Build history of the part. All positions in model axes, mm. A direction names the side the tool comes from. Give positions to 0.01 mm unless a question says otherwise; leave off trailing zeros. Order: outer loops, then holes, each group sorted by start corner. A loop starts at its lowest first (then second) coordinate and runs counter-clockwise, first axis right, second up. Notation, with made-up numbers: M 48,3 L 82,3 A25 ccw 82,26 Z; hole C 69,-8.75 d5. An arc over 180 degrees is marked long. One line per item, written item: value.
from build123d import *

# Parameters (mm, degrees)
SZKIC1_W                    = 121
SZKIC1_H                    = 24
SZKIC1_R                    = 7.5
DODANIE_WYCI_GNI_CIE1_DEPTH = 3
SZKIC2_W                    = 121
SZKIC2_H                    = 24
SZKIC2_W_2                  = 39
SZKIC2_H_2                  = 20
DODANIE_WYCI_GNI_CIE2_DEPTH = 2
SZKIC3_W                    = 10
SZKIC3_H                    = 21
SZKIC3_W_2                  = 18
DODANIE_WYCI_GNI_CIE3_DEPTH = 5
SZKIC5_W                    = 18
SZKIC5_H                    = 9
DODANIE_WYCI_GNI_CIE4_DEPTH = 2.5
WYTNIJ_WYCI_GNI_CIE1_REACH  = 103.983
SZKIC6_R                    = 1.75
WYTNIJ_WYCI_GNI_CIE2_START  = -1.5
SZKIC7_R                    = 3.75
SZKIC7_R_2                  = 1.75
WYTNIJ_WYCI_GNI_CIE2_DEPTH  = 1.5
WYTNIJ_WYCI_GNI_CIE4_DEPTH  = 1.5
ZAOKR_GLENIE1_R             = 1.5
SZKIC10_W                   = 10
SZKIC10_H                   = 7.5
SZKIC10_W_2                 = 18
WYTNIJ_WYCI_GNI_CIE5_DEPTH  = 0.2
SZKIC11_W                   = 121
SZKIC11_H                   = 1.5
DODANIE_WYCI_GNI_CIE5_DEPTH = 45
SFAZOWANIE1_SIZE            = 1
SFAZOWANIE2_SIZE            = 1


with BuildPart() as part:
    # Szkic1 → Dodanie-wyciągnięcie1 (new body)
    with BuildSketch(Plane.XY):
        with Locations((40, 0)):
            Rectangle(SZKIC1_W, SZKIC1_H)
        Circle(SZKIC1_R, mode=Mode.SUBTRACT)
        with Locations((80, 0)):
            Circle(SZKIC1_R, mode=Mode.SUBTRACT)
    extrude(amount=DODANIE_WYCI_GNI_CIE1_DEPTH)

    # Szkic2 → Dodanie-wyciągnięcie2 (add)
    with BuildSketch(Plane.XY.offset(3)):
        with Locations((40, 0)):
            Rectangle(SZKIC2_W, SZKIC2_H)
        with Locations((9, 0)):
            Rectangle(SZKIC2_W_2, SZKIC2_H_2, mode=Mode.SUBTRACT)
        with Locations((71, 0)):
            Rectangle(SZKIC2_W_2, SZKIC2_H_2, mode=Mode.SUBTRACT)
    extrude(amount=DODANIE_WYCI_GNI_CIE2_DEPTH)

    # Szkic3 → Dodanie-wyciągnięcie3 (add)
    with BuildSketch(Plane.XY.offset(5)):
        with Locations((-15.5, 0)):
            Rectangle(SZKIC3_W, SZKIC3_H)
        with Locations((40, 0)):
            Rectangle(SZKIC3_W_2, SZKIC3_H)
        with Locations((95.5, 0)):
            Rectangle(SZKIC3_W, SZKIC3_H)
    extrude(amount=DODANIE_WYCI_GNI_CIE3_DEPTH)

    # Szkic5 → Dodanie-wyciągnięcie4 (add)
    with BuildSketch(Plane.XY.offset(10)):
        Polygon((-20.5, 10.5), (-10.5, 10.5), (-10.5, 1.5), (-19, 1.5), (-19, -1.5), (-10.5, -1.5), (-10.5, -10.5), (-20.5, -10.5), align=None)
        Polygon((90.5, -1.5), (99, -1.5), (99, 1.5), (90.5, 1.5), (90.5, 10.5), (100.5, 10.5), (100.5, -10.5), (90.5, -10.5), align=None)
        with Locations((40, -6)):
            Rectangle(SZKIC5_W, SZKIC5_H)
        with Locations((40, 6)):
            Rectangle(SZKIC5_W, SZKIC5_H)
    extrude(amount=DODANIE_WYCI_GNI_CIE4_DEPTH)

    # Szkic6 → Wytnij-wyciągnięcie1 (cut, up to next)
    with BuildSketch(Plane.XY.offset(12.5), mode=Mode.PRIVATE) as wytnij_wyci_gni_cie1_sk1:
        with Locations((-14.5, 5.45)):
            Circle(SZKIC6_R)
    wytnij_wyci_gni_cie1_tool1 = extrude(wytnij_wyci_gni_cie1_sk1.sketch, amount=-WYTNIJ_WYCI_GNI_CIE1_REACH, mode=Mode.PRIVATE) & part.part
    # Szkic6 → Wytnij-wyciągnięcie1 (cut, up to next)
    with BuildSketch(Plane.XY.offset(12.5), mode=Mode.PRIVATE) as wytnij_wyci_gni_cie1_sk2:
        with Locations((34.5, 5.45)):
            Circle(SZKIC6_R)
    wytnij_wyci_gni_cie1_tool2 = extrude(wytnij_wyci_gni_cie1_sk2.sketch, amount=-WYTNIJ_WYCI_GNI_CIE1_REACH, mode=Mode.PRIVATE) & part.part
    # Szkic6 → Wytnij-wyciągnięcie1 (cut, up to next)
    with BuildSketch(Plane.XY.offset(12.5), mode=Mode.PRIVATE) as wytnij_wyci_gni_cie1_sk3:
        with Locations((34.5, -5.45)):
            Circle(SZKIC6_R)
    wytnij_wyci_gni_cie1_tool3 = extrude(wytnij_wyci_gni_cie1_sk3.sketch, amount=-WYTNIJ_WYCI_GNI_CIE1_REACH, mode=Mode.PRIVATE) & part.part
    # Szkic6 → Wytnij-wyciągnięcie1 (cut, up to next)
    with BuildSketch(Plane.XY.offset(12.5), mode=Mode.PRIVATE) as wytnij_wyci_gni_cie1_sk4:
        with Locations((-14.5, -5.45)):
            Circle(SZKIC6_R)
    wytnij_wyci_gni_cie1_tool4 = extrude(wytnij_wyci_gni_cie1_sk4.sketch, amount=-WYTNIJ_WYCI_GNI_CIE1_REACH, mode=Mode.PRIVATE) & part.part
    # Szkic6 → Wytnij-wyciągnięcie1 (cut, up to next)
    with BuildSketch(Plane.XY.offset(12.5), mode=Mode.PRIVATE) as wytnij_wyci_gni_cie1_sk5:
        with Locations((45.5, 5.45)):
            Circle(SZKIC6_R)
    wytnij_wyci_gni_cie1_tool5 = extrude(wytnij_wyci_gni_cie1_sk5.sketch, amount=-WYTNIJ_WYCI_GNI_CIE1_REACH, mode=Mode.PRIVATE) & part.part
    # Szkic6 → Wytnij-wyciągnięcie1 (cut, up to next)
    with BuildSketch(Plane.XY.offset(12.5), mode=Mode.PRIVATE) as wytnij_wyci_gni_cie1_sk6:
        with Locations((45.5, -5.45)):
            Circle(SZKIC6_R)
    wytnij_wyci_gni_cie1_tool6 = extrude(wytnij_wyci_gni_cie1_sk6.sketch, amount=-WYTNIJ_WYCI_GNI_CIE1_REACH, mode=Mode.PRIVATE) & part.part
    # Szkic6 → Wytnij-wyciągnięcie1 (cut, up to next)
    with BuildSketch(Plane.XY.offset(12.5), mode=Mode.PRIVATE) as wytnij_wyci_gni_cie1_sk7:
        with Locations((94.5, -5.45)):
            Circle(SZKIC6_R)
    wytnij_wyci_gni_cie1_tool7 = extrude(wytnij_wyci_gni_cie1_sk7.sketch, amount=-WYTNIJ_WYCI_GNI_CIE1_REACH, mode=Mode.PRIVATE) & part.part
    # Szkic6 → Wytnij-wyciągnięcie1 (cut, up to next)
    with BuildSketch(Plane.XY.offset(12.5), mode=Mode.PRIVATE) as wytnij_wyci_gni_cie1_sk8:
        with Locations((94.5, 5.45)):
            Circle(SZKIC6_R)
    wytnij_wyci_gni_cie1_tool8 = extrude(wytnij_wyci_gni_cie1_sk8.sketch, amount=-WYTNIJ_WYCI_GNI_CIE1_REACH, mode=Mode.PRIVATE) & part.part
    add(wytnij_wyci_gni_cie1_tool1.solids().sort_by_distance((-14.5, 5.45, 12.5))[0], mode=Mode.SUBTRACT)
    add(wytnij_wyci_gni_cie1_tool2.solids().sort_by_distance((34.5, 5.45, 12.5))[0], mode=Mode.SUBTRACT)
    add(wytnij_wyci_gni_cie1_tool3.solids().sort_by_distance((34.5, -5.45, 12.5))[0], mode=Mode.SUBTRACT)
    add(wytnij_wyci_gni_cie1_tool4.solids().sort_by_distance((-14.5, -5.45, 12.5))[0], mode=Mode.SUBTRACT)
    add(wytnij_wyci_gni_cie1_tool5.solids().sort_by_distance((45.5, 5.45, 12.5))[0], mode=Mode.SUBTRACT)
    add(wytnij_wyci_gni_cie1_tool6.solids().sort_by_distance((45.5, -5.45, 12.5))[0], mode=Mode.SUBTRACT)
    add(wytnij_wyci_gni_cie1_tool7.solids().sort_by_distance((94.5, -5.45, 12.5))[0], mode=Mode.SUBTRACT)
    add(wytnij_wyci_gni_cie1_tool8.solids().sort_by_distance((94.5, 5.45, 12.5))[0], mode=Mode.SUBTRACT)

    # Szkic7 → Wytnij-wyciągnięcie2 (cut)
    # profile 1 of 4: a face of its own
    with BuildSketch(Plane(origin=(0, 0, 0), x_dir=(-1, 0, 0), z_dir=(0, 0, -1)).offset(WYTNIJ_WYCI_GNI_CIE2_START)):
        with Locations((14.5, -5.45)):
            Circle(SZKIC7_R)
        with Locations(Location((14.5, -5.45, 0), (0, 0, 180))):
            Circle(SZKIC7_R_2, mode=Mode.SUBTRACT)
    # profile 2 of 4: a face of its own
    with BuildSketch(Plane(origin=(0, 0, 0), x_dir=(-1, 0, 0), z_dir=(0, 0, -1)).offset(WYTNIJ_WYCI_GNI_CIE2_START)):
        with Locations((14.5, 5.45)):
            Circle(SZKIC7_R)
        with Locations(Location((14.5, 5.45, 0), (0, 0, 180))):
            Circle(SZKIC7_R_2, mode=Mode.SUBTRACT)
    # profile 3 of 4: a face of its own
    with BuildSketch(Plane(origin=(0, 0, 0), x_dir=(-1, 0, 0), z_dir=(0, 0, -1)).offset(WYTNIJ_WYCI_GNI_CIE2_START)):
        with Locations((-94.5, -5.45)):
            Circle(SZKIC7_R)
        with Locations(Location((-94.5, -5.45, 0), (0, 0, 180))):
            Circle(SZKIC7_R_2, mode=Mode.SUBTRACT)
    # profile 4 of 4: a face of its own
    with BuildSketch(Plane(origin=(0, 0, 0), x_dir=(-1, 0, 0), z_dir=(0, 0, -1)).offset(WYTNIJ_WYCI_GNI_CIE2_START)):
        with Locations((-94.5, 5.45)):
            Circle(SZKIC7_R)
        with Locations(Location((-94.5, 5.45, 0), (0, 0, 180))):
            Circle(SZKIC7_R_2, mode=Mode.SUBTRACT)
    extrude(amount=WYTNIJ_WYCI_GNI_CIE2_DEPTH, mode=Mode.SUBTRACT)

    # Szkic9 → Wytnij-wyciągnięcie4 (cut)
    with BuildSketch(Plane(origin=(0, 0, 0), x_dir=(-1, 0, 0), z_dir=(0, 0, -1))):
        with BuildLine():
            Line((-40.883453672, 7.95), (-39.116546328, 7.95))
            ThreePointArc((-39.116546328, 7.95), (-29.25, 5.45), (-39.116546328, 2.95))
            Line((-39.116546328, 2.95), (-40.883453672, 2.95))
            ThreePointArc((-40.883453672, 2.95), (-50.75, 5.45), (-40.883453672, 7.95))
        make_face()
        with BuildLine():
            Line((-40.883453672, -7.95), (-39.116546328, -7.95))
            ThreePointArc((-39.116546328, -7.95), (-29.25, -5.45), (-39.116546328, -2.95))
            Line((-39.116546328, -2.95), (-40.883453672, -2.95))
            ThreePointArc((-40.883453672, -2.95), (-50.75, -5.45), (-40.883453672, -7.95))
        make_face()
    extrude(amount=-WYTNIJ_WYCI_GNI_CIE4_DEPTH, mode=Mode.SUBTRACT)

    # Zaokrąglenie1
    zaokr_glenie1_edges = [part.edges().sort_by_distance(p)[0] for p in [
        (39.116546328, -7.95, 0.75),
        (39.116546328, -2.95, 0.75),
        (40.883453672, -2.95, 0.75),
        (40.883453672, -7.95, 0.75),
        (39.116546328, 2.95, 0.75),
        (39.116546328, 7.95, 0.75),
        (40.883453672, 7.95, 0.75),
        (40.883453672, 2.95, 0.75),
    ]]
    fillet(zaokr_glenie1_edges, radius=ZAOKR_GLENIE1_R)

    # Szkic10 → Wytnij-wyciągnięcie5 (cut)
    with BuildSketch(Plane(origin=(0, 10.5, 0), x_dir=(1, 0, 0), z_dir=(0, 1, 0))):
        with Locations((-15.5, -8.75)):
            Rectangle(SZKIC10_W, SZKIC10_H)
        with Locations((40, -8.75)):
            Rectangle(SZKIC10_W_2, SZKIC10_H)
        with Locations((95.5, -8.75)):
            Rectangle(SZKIC10_W, SZKIC10_H)
    extrude(amount=-WYTNIJ_WYCI_GNI_CIE5_DEPTH, mode=Mode.SUBTRACT)

    # Szkic11 → Dodanie-wyciągnięcie5 (add)
    with BuildSketch(Plane.XY.offset(5)):
        with Locations((40, -11.25)):
            Rectangle(SZKIC11_W, SZKIC11_H)
    extrude(amount=DODANIE_WYCI_GNI_CIE5_DEPTH)

    # Sfazowanie1
    sfazowanie1_edges = [part.edges().sort_by_distance(p)[0] for p in [
        (40, -12, 0),
        (-20.5, 0, 0),
        (40, 12, 0),
        (100.5, 0, 0),
    ]]
    chamfer(sfazowanie1_edges, length=SFAZOWANIE1_SIZE)

    # Sfazowanie2
    sfazowanie2_edges = [part.edges().sort_by_distance(p)[0] for p in [
        (100.5, -12, 25.5),
        (-20.5, -12, 25.5),
        (-20.5, 12, 3),
        (100.5, 12, 3),
    ]]
    chamfer(sfazowanie2_edges, length=SFAZOWANIE2_SIZE)


solid = part.part
1) Drill centre lines: probe 1 along Y at (x, z) = (32, 42.5); probe 2 along Z at (x, y) = (57, -4.75); probe 3 along Z at (x, y) = (92.5, 9). Where is each one in solid material? Low to high. Write a range as from..to.
Check values:
probe 1: -12..-10.5
probe 2: 0..3
probe 3: 0..12.5
2) Saw through at C-C, the plane z = 44. Write the cut outline in (x, y), then the cut area to 4 significant figures.
Check values:
outline: M -20.5,-11 L -19.5,-12 L 99.5,-12 L 100.5,-11 L 100.5,-10.5 L -20.5,-10.5 Z
area: 180.5 mm^2
3) Saw through at B-B, the plane x = 94.5. Give the number of separate pieces and of enclosed holes in the cut face, then the cut area to 4 significant figures.
Check values:
separate pieces: 3
enclosed holes: 0
area: 235.5 mm^2
4) Mould opens along X. For faces 1 (the face through (-12.883, -6.12, 7.077)), 2 (the face through (100.5, -2, 9)), 3 (the face through (40, -6, 12.5)) say: released by +X, released by -X, zero draft, split by the parting line, or undercut.
Check values:
face 1: undercut
face 2: released by +X
face 3: zero draft
5) Pin check, flat tips, straight feed: pin 1 (8.5 mm diameter, centred on x = 94.5, y = 5.45, fed in from -Z); pin 2 (4 mm diameter, centred on x = -14.5, y = -5.45, fed in from +Z); pin 3 (5 mm diameter, centred on x = 44.5, y = 3.5, fed in from -Z); pin 4 (10 mm diameter, centred on x = 45.5, z = 34, fed in from +Y). Stop position of each tip, or through.
Check values:
pin 1: z = 0
pin 2: z = 12.5
pin 3: z = 1.5
pin 4: y = -10.5
6) Saw through at A-A, the plane x = 80. Write the cut outline in (y, z).
Check values:
outline: M -12,1 L -11,0 L -7.5,0 L -7.5,3 L -10,3 L -10,5 L -10.5,5 L -10.5,50 L -12,50 Z; M 7.5,0 L 11,0 L 12,1 L 12,5 L 10,5 L 10,3 L 7.5,3 Z
7) Tool access for faces 4 (the face through (49, 0, 9)), 5 (the face through (39, 12, 3)), 6 (the face through (40, -5, 1.5)), 7 (the face through (90.5, 0, 8)): list every direction of +Z, -Z, +X, -X, +Y, -Y with a clear straight run to the whole face (end or side of a thin tool).
Check values:
face 4: +Z, +Y
face 5: +Z, -Z, +X, -X, +Y
face 6: -Z
face 7: +Z
